Verification items for the finished model (mm, model axes). Coordinates: 2 decimals unless noted, no trailing zeros. Order: outer loops, then holes, each group sorted by start corner. A loop starts at its lowest first (then second) coordinate and runs counter-clockwise, first axis right, second up. Notation, with made-up numbers: M 56,-5 L 108,-5 A27 cw 108,30 Z; hole C 1.5,31.25 d3. An arc over 180 degrees is marked long. Return JSON: item names as keys, results as strings.
```python
from build123d import *

# Parameters (mm, degrees)
BOSS_EXTRUDE1_DEPTH = 2336.8
SKETCH3_R           = 25.4
BOSS_EXTRUDE2_DEPTH = 304.8
SKETCH4_R           = 12.7
CUT_EXTRUDE2_DEPTH  = 16.51


with BuildPart() as part:
    # Sketch1 → Boss-Extrude1 (new body)
    with BuildSketch(Plane(origin=(0, 0, 0), x_dir=(0, 0, -1), z_dir=(1, 0, 0))):
        Polygon((59.182, 67.564), (59.182, 76.2), (0, 76.2), (0, 67.564), (27.432, 67.564), (27.432, 8.636), (0, 8.636), (0, 0), (59.182, 0), (59.182, 8.636), (31.75, 8.636), (31.75, 67.564), align=None)
    extrude(amount=BOSS_EXTRUDE1_DEPTH)

    # Sketch3 → Boss-Extrude2 (add)
    with BuildSketch(Plane(origin=(0, 76.2, 0), x_dir=(1, 0, 0), z_dir=(0, 1, 0))):
        with Locations(Location((2184.4, 29.591, 0), (0, 0, 90))):
            Circle(SKETCH3_R)
    extrude(amount=BOSS_EXTRUDE2_DEPTH)

    # Sketch4 → Cut-Extrude2 (cut)
    with BuildSketch(Plane.XY.offset(-31.75)):
        with Locations(Location((787.4, 38.1, 0), (0, 0, 180))):
            Circle(SKETCH4_R)
    extrude(amount=CUT_EXTRUDE2_DEPTH, mode=Mode.SUBTRACT)


solid = part.part
```
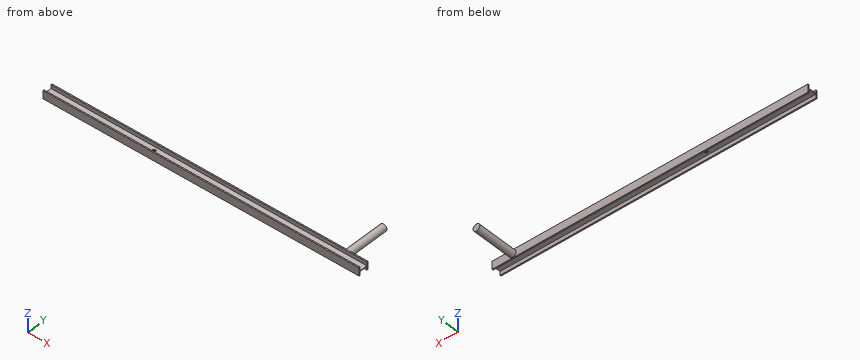
Q1. Cross-section at C-C, the plane y = 304. Record the boundary of the cut face in (x, z).
Values:
{"outline": "C 2184.4,-29.59 d50.8"}
Q2. Material ranges on line 1 along Y through (x, z) = (787.4, -28.8); line 2 along Y through (x, z) = (1871.5, -44.5); line 3 along X through (y, z) = (38.1, -30.2), recorded low to high.
Values:
{"line 1": "0 to 25.4, 50.8 to 76.2", "line 2": "0 to 8.64, 67.56 to 76.2", "line 3": "0 to 774.7, 800.1 to 2336.8"}
Q3. Cross-section at B-B, the plane x = 2184.4. Record the boundary of the cut face in (y, z), and give its area (3 significant figures).
Values:
{"outline": "M 0,-59.18 L 8.64,-59.18 L 8.64,-31.75 L 67.56,-31.75 L 67.56,-59.18 L 76.2,-59.18 L 76.2,-54.99 L 381,-54.99 L 381,-4.19 L 76.2,-4.19 L 76.2,0 L 67.56,0 L 67.56,-27.43 L 8.64,-27.43 L 8.64,0 L 0,0 Z", "area": "16,800 mm^2"}
Q4. Go/stop test with flat-tipped pins: pin 1 (6 mm diameter, centred on y = 225.5, z = -32, fed in from -X); pin 2 (13.5 mm diameter, centred on x = 1471.5, z = -14.5, fed in from +Y). Record where each tip stops, or that it passes through.
Values:
{"pin 1": "x = 2159", "pin 2": "y = 76.2"}
Q5. Cross-section at A-A, the plane x = 897. Record the boundary of the cut face in (y, z), and give its area (3 significant figures).
Values:
{"outline": "M 0,-59.18 L 8.64,-59.18 L 8.64,-31.75 L 67.56,-31.75 L 67.56,-59.18 L 76.2,-59.18 L 76.2,0 L 67.56,0 L 67.56,-27.43 L 8.64,-27.43 L 8.64,0 L 0,0 Z", "area": "1,280 mm^2"}
